Part model, mm, in its own coordinate system. Round coordinates to 2 decimals unless told otherwise and drop trailing zeros. Write each loop counter-clockwise with the first axis right and the second up, starting at its lowest first coordinate (ties: lowest second). Pieces come first, ordered by that corner, then holes. Notation, with made-up numbers: M 67.25,-2.5 L 87.25,-2.5 A10 cw 87.25,3.5 Z; hole C -16.75,9 d5. An arc over 180 degrees is marked long. Answer as a JSON object with one key per item and string values. Group by question number.
1. Drop flat-ended pins along their axis: pin 1 (8 mm diameter, centred on y = 35, z = 116.5, fed in from +X); pin 2 (12 mm diameter, centred on x = -27, y = 13, fed in from -Z); pin 3 (1 mm diameter, centred on y = 30.5, z = 113, fed in from +X); pin 4 (6 mm diameter, centred on y = 22, z = 53, fed in from +X). Give the stop position or say it passes through.
2. Band-saw the part on A-A, the plane z = 46. Write the cut outline in (x, y).
3. Drill centre lines: line 1 (X direction, y = 36.5, z = 103); line 2 (X direction, y = 33.5, z = 76); line 3 (Y direction, x = -32, z = 88). Where is each one in solid material? Low to high. Write a range as from..to.
4. Band-saw the part on C-C, the plane x = -17.5. Write the cut outline in (y, z), plus the area to 3 significant figures.
5. Band-saw the part on B-B, the plane y = 31. Write the cut outline in (x, z), plus the area to 3 significant figures.
from build123d import *

# Parameters (mm, degrees)
F1_DEPTH = 150
F3_DEPTH = 140


with BuildPart() as f1:
    # F0 (on Top) → F1 (new body)
    with BuildSketch(Plane.XY):
        with BuildLine():
            Line((-35.705528, 49.347393), (-67.291312, 49.347393))
            ThreePointArc((-67.291312, 49.347393), (-68.705525, 48.761607), (-69.291312, 47.347393))
            Line((-69.291312, 47.347393), (-69.291312, 3.347397))
            ThreePointArc((-69.291312, 3.347397), (-68.705525, 1.933183), (-67.291312, 1.347397))
            Line((-67.291312, 1.347397), (9.537109, 1.347397))
            ThreePointArc((9.537109, 1.347397), (11.384868, 2.58203), (10.951323, 4.76161))
            Line((10.951323, 4.76161), (-32.169994, 47.882927))
            ThreePointArc((-32.169994, 47.882927), (-33.792111, 48.966791), (-35.705528, 49.347393))
        make_face()
        with BuildLine():
            ThreePointArc((-65.291314, 44.347395), (-64.99842, 45.054502), (-64.291314, 45.347395))
            Line((-64.291314, 45.347395), (-36.119741, 45.347395))
            ThreePointArc((-36.119741, 45.347395), (-35.354374, 45.195154), (-34.705527, 44.761609))
            Line((-34.705527, 44.761609), (3.00158, 7.054502))
            ThreePointArc((3.00158, 7.054502), (3.218352, 5.964712), (2.294473, 5.347395))
            Line((2.294473, 5.347395), (-64.291314, 5.347395))
            ThreePointArc((-64.291314, 5.347395), (-64.99842, 5.640288), (-65.291314, 6.347395))
            Line((-65.291314, 6.347395), (-65.291314, 44.347395))
        make_face(mode=Mode.SUBTRACT)
    extrude(amount=F1_DEPTH)


with BuildPart() as f3:
    # F2 (on Top) → F3 (new body)
    with BuildSketch(Plane.XY):
        with BuildLine():
            Line((-37.362381, 41.347396), (-60.291314, 41.347396))
            ThreePointArc((-60.291314, 41.347396), (-60.998421, 41.054502), (-61.291314, 40.347396))
            Line((-61.291314, 40.347396), (-61.291314, 10.347394))
            ThreePointArc((-61.291314, 10.347394), (-60.998421, 9.640288), (-60.291314, 9.347394))
            Line((-60.291314, 9.347394), (-7.36238, 9.347394))
            ThreePointArc((-7.36238, 9.347394), (-6.4385, 9.964711), (-6.655273, 11.054501))
            Line((-6.655273, 11.054501), (-36.655274, 41.054502))
            ThreePointArc((-36.655274, 41.054502), (-36.979698, 41.271275), (-37.362381, 41.347396))
        make_face()
    extrude(amount=F3_DEPTH)


solid = f3.part
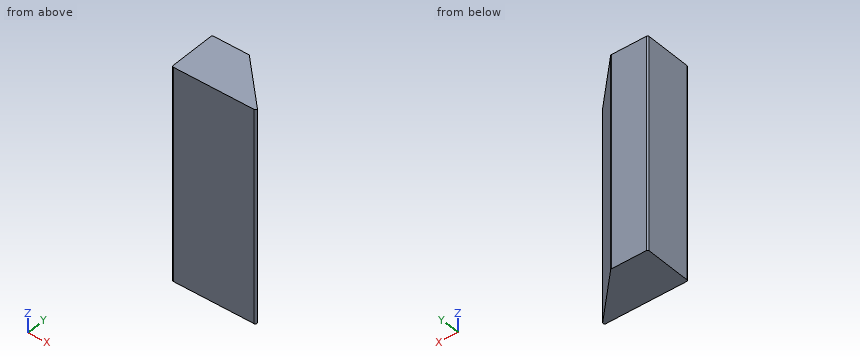
Worked answers:
{
 "1": {"pin 1": "stops at x = -26.6", "pin 2": "stops at z = 0", "pin 3": "stops at x = -25.6", "pin 4": "stops at x = -14.6"},
 "2": {"outline": "M -61.29,10.35 A1 ccw -60.29,9.35 L -7.36,9.35 A1 ccw -6.66,11.05 L -36.66,41.05 A1 ccw -37.36,41.35 L -60.29,41.35 A1 ccw -61.29,40.35 Z"},
 "3": {"line 1": "x = -61.29..-32.1", "line 2": "x = -61.29..-29.1", "line 3": "y = 9.35..36.4"},
 "4": {"outline": "M 9.35,0 L 21.9,0 L 21.9,140 L 9.35,140 Z", "area": "1,760 mm^2"},
 "5": {"outline": "M -61.29,0 L -26.6,0 L -26.6,140 L -61.29,140 Z", "area": "4,860 mm^2"}
}
